Source: CAD feature listing. Evaluate the final solid. Frame: model axes, mm. Face numbers are marked on the shaded views. A direction names the side the tool comes from. Give positions to 0.01 mm unless a question says otherwise; leave off trailing zeros. Order: outer loops, then holes, each group sorted by start corner. A loop starts at its lowest first (then second) coordinate and runs counter-clockwise, first axis right, second up. Notation, with made-up numbers: (78.5, 78.25) - (102.5, 78.25) arc R27 cw to (102.5, 114.25) - close; hole circle Ø6 at (60.25, 57). An arc over 180 degrees is marked (long way). Write each question's results on one line, items separated by ' | '. Start each with the question number.
Item 1: Mould query, pull axis Z, two halves, no side actions, for the marked faces 1, 2 and 3. Classes: released by +Z, released by -Z, zero draft, split by the parting line, or undercut.
Item 2: Set-up query: the marked faces 4, 5 and 6. Return all of +Z, -Z, +X, -X, +Y, -Y with unobstructed straight access to the full face (end or side cutting, diameter ignored); none if empty.
Item 3: Section A-A on x = -40. Output: boundary loops of the cut face in (y, z), and give its area (3 significant figures).
Item 4: Section D-D on z = -4. Output: boundary loops of the cut face in (x, y).
Item 5: Line query: line 1 along Y through (x, z) = (25.4, -7.5); line 2 along X through (y, z) = (-9.5, 13); line 3 along X through (y, z) = (-21.5, 41.5). Output: solid intervals per line, ascending.
Item 6: Section B-B on x = 25.4. Output: boundary loops of the cut face in (y, z), and give its area (3 significant figures).
Item 7: Contact query for flat-ended pins moving along their axis: pin 1 Ø18.5 at (y, z) = (-1, 16) entering from -X; pin 2 Ø14.5 at (x, y) = (0, 0) entering from -Z; pin 3 Ø5.5 at (x, y) = (-25.4, 8.128) entering from +Z. Output: stop coordinate, or through.
Item 8: Section C-C on x = -16.5. Output: boundary loops of the cut face in (y, z), and give its area (3 significant figures).
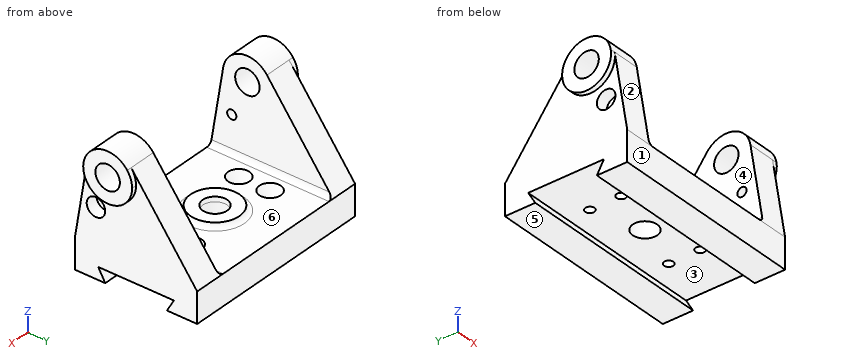
```python
from build123d import *

# Parameters (mm, degrees)
F0_R            = 6.35
F1_DEPTH        = 50.8
F2_DEPTH        = 53.34
F3_DEPTH        = 36.576
F5_D            = 4.7752
F5_CSINK_D      = 11.176
F5_CSINK_ANGLE  = 60
F4_R            = 6.35
F6_DEPTH        = 25.4
F4_R_2          = 12.7
F7_DEPTH        = 2.54
F8_R            = 2.53999
F10_D           = 4.7752
F10_DEPTH       = 25.4
F10_CBORE_D     = 9.652
F10_CBORE_DEPTH = 6.35
F10_TIP         = 1.434614814
F12_D           = 4.7752
F12_DEPTH       = 25.4
F12_CBORE_D     = 9.652
F12_CBORE_DEPTH = 6.35
F12_TIP         = 1.434614814


# Not quite as in the source:
# - a fillet or chamfer is up to 0.001 mm smaller than in the source, because OpenCascade refuses the exact size


with BuildPart() as f1:
    # F0 (on Right) → F1 (new body, symmetric)
    with BuildSketch(Plane.YZ):
        with BuildLine():
            ThreePointArc((-25.2359570421, 40.1346451877), (-13.7206237225, 25.44107717), (0, 38.1))
            ThreePointArc((0, 38.1), (-0.6517221148, 42.1160926284), (-2.54, 45.72))
            ThreePointArc((-2.54, 45.72), (-15.7348542076, 50.4320582199), (-25.2359570421, 40.1346451877))
        make_face()
        with Locations((-12.7, 38.1)):
            Circle(F0_R, mode=Mode.SUBTRACT)
        with BuildLine():
            ThreePointArc((-2.54, 45.72), (-0.6517221148, 42.1160926284), (0, 38.1))
            ThreePointArc((0, 38.1), (-13.7206237225, 25.44107717), (-25.2359570421, 40.1346451877))
            Line((-25.2359570421, 40.1346451877), (-31.75, 0))
            Line((-31.75, 0), (31.75, 0))
            Line((31.75, 0), (-2.54, 45.72))
        make_face()
        Polygon((31.75, -15.748), (31.75, 0), (-31.75, 0), (-31.75, -15.748), (-16.002, -15.748), (-19.6681742094, -9.398), (19.6681742094, -9.398), (16.002, -15.748), align=None)
    extrude(amount=F1_DEPTH, both=True)

    # F0 (on Right) → F2 (join, symmetric)
    with BuildSketch(Plane.YZ):
        with BuildLine():
            ThreePointArc((-25.2359570421, 40.1346451877), (-13.7206237225, 25.44107717), (0, 38.1))
            ThreePointArc((0, 38.1), (-0.6517221148, 42.1160926284), (-2.54, 45.72))
            ThreePointArc((-2.54, 45.72), (-15.7348542076, 50.4320582199), (-25.2359570421, 40.1346451877))
        make_face()
        with Locations((-12.7, 38.1)):
            Circle(F0_R, mode=Mode.SUBTRACT)
    extrude(amount=F2_DEPTH, both=True)

    # F0 (on Right) → F3 (cut, symmetric)
    with BuildSketch(Plane.YZ):
        with BuildLine():
            ThreePointArc((-2.54, 45.72), (-0.6517221148, 42.1160926284), (0, 38.1))
            ThreePointArc((0, 38.1), (-13.7206237225, 25.44107717), (-25.2359570421, 40.1346451877))
            Line((-25.2359570421, 40.1346451877), (-31.75, 0))
            Line((-31.75, 0), (31.75, 0))
            Line((31.75, 0), (-2.54, 45.72))
        make_face()
        with BuildLine():
            ThreePointArc((-25.2359570421, 40.1346451877), (-13.7206237225, 25.44107717), (0, 38.1))
            ThreePointArc((0, 38.1), (-0.6517221148, 42.1160926284), (-2.54, 45.72))
            ThreePointArc((-2.54, 45.72), (-15.7348542076, 50.4320582199), (-25.2359570421, 40.1346451877))
        make_face()
        with Locations((-12.7, 38.1)):
            Circle(F0_R, mode=Mode.SUBTRACT)
    extrude(amount=F3_DEPTH, both=True, mode=Mode.SUBTRACT)

    # F5 (through all)
    with Locations(Plane.XY):
        with Locations((-25.4, 8.128), (-25.4, -8.128), (25.4, 8.128), (25.4, -8.128)):
            CounterSinkHole(F5_D / 2, F5_CSINK_D / 2, counter_sink_angle=F5_CSINK_ANGLE)

    # F4 (on face) → F6 (cut)
    with BuildSketch(Plane.XY):
        Circle(F4_R)
    extrude(amount=-F6_DEPTH, mode=Mode.SUBTRACT)

    # F4 (on face) → F7 (join)
    with BuildSketch(Plane.XY):
        Circle(F4_R_2)
        Circle(F4_R, mode=Mode.SUBTRACT)
    extrude(amount=F7_DEPTH)

    # F8 (radius 2.54 in the source; OpenCascade refuses exactly that, so slightly less here)
    f8_edges = [f1.edges().sort_by_distance(p)[0] for p in [
        (-12.7, 0, 0),
        (36.576, 0, 0),
        (-36.576, 0, 0),
    ]]
    fillet(f8_edges, radius=F8_R)

    # F10
    with Locations(Plane.YZ.offset(50.8)):
        with Locations((-20.828, 19.05)):
            CounterBoreHole(F10_D / 2, F10_CBORE_D / 2, F10_CBORE_DEPTH, depth=F10_DEPTH)
            with Locations((0, 0, -(F10_DEPTH + F10_TIP / 2))):  # 118° drill point
                Cone(0, F10_D / 2, F10_TIP, mode=Mode.SUBTRACT)

    # F12
    with Locations(Plane(origin=(-50.8, 0, 0), x_dir=(0, -1, 0), z_dir=(-1, 0, 0))):
        with Locations((20.828, 19.05)):
            CounterBoreHole(F12_D / 2, F12_CBORE_D / 2, F12_CBORE_DEPTH, depth=F12_DEPTH)
            with Locations((0, 0, -(F12_DEPTH + F12_TIP / 2))):  # 118° drill point
                Cone(0, F12_D / 2, F12_TIP, mode=Mode.SUBTRACT)


solid = f1.part
```
Evaluation:
1) face 1: zero draft | face 2: released by +Z | face 3: undercut
2) face 4: +Z, +Y, -Y | face 5: -Z, +X, -X, +Y, -Y | face 6: +Z
3) outline: (-31.75, -15.75) - (-16, -15.75) - (-19.67, -9.4) - (19.67, -9.4) - (16, -15.75) - (31.75, -15.75) - (31.75, 0) - (-2.54, 45.72) arc R12.7 ccw to (-25.24, 40.13) - (-31.75, 0) - close; hole circle Ø4.78 at (-20.83, 19.05); hole circle Ø12.7 at (-12.7, 38.1) | area: 2,650 mm^2
4) outline: (-50.8, -31.75) - (50.8, -31.75) - (50.8, 31.75) - (-50.8, 31.75) - close; hole circle Ø6.56 at (-25.4, -8.13); hole circle Ø6.56 at (-25.4, 8.13); hole circle Ø12.7 at (0, 0); hole circle Ø6.56 at (25.4, -8.13); hole circle Ø6.56 at (25.4, 8.13)
5) line 1: y = -31.75 to -10.52, -5.74 to 5.74, 10.52 to 31.75 | line 2: x = -50.8 to -36.58, 36.58 to 50.8 | line 3: x = -53.34 to -36.58, 36.58 to 53.34
6) outline: (-31.75, -15.75) - (-16, -15.75) - (-19.67, -9.4) - (-10.52, -9.4) - (-10.52, -5.54) - (-13.72, 0) - (-31.75, 0) - close; (-5.74, -9.4) - (5.74, -9.4) - (5.74, -5.54) - (2.54, 0) - (-2.54, 0) - (-5.74, -5.54) - close; (10.52, -9.4) - (19.67, -9.4) - (16, -15.75) - (31.75, -15.75) - (31.75, 0) - (13.72, 0) - (10.52, -5.54) - close | area: 648 mm^2
7) pin 1: stops at x = -50.8 | pin 2: stops at z = -9.4 | pin 3: stops at z = -4.92
8) outline: (-31.75, -15.75) - (-16, -15.75) - (-19.67, -9.4) - (19.67, -9.4) - (16, -15.75) - (31.75, -15.75) - (31.75, 0) - (-31.75, 0) - close | area: 773 mm^2
